Can you work these out from the model? Positions are in its coordinate system, mm. Face numbers are marked on the shaded views. Coordinates: 2 decimals unless noted, no trailing zeros. Loops run counter-clockwise (first coordinate to the right, second up) from the corner with the lowest first, then second, coordinate; pieces in that order, holes last. Notation, with made-up numbers: (61, -26) -> (95, -26) arc R32 cw to (95, 12) -> close; hole circle Ø9 at (39, -15). An arc over 180 degrees is marked (long way). Use one line per item in the form item = value. Start each with the question number.
(1) Imagine slicing it at A-A (z = 0). List the corners of the cut face in (x, y) for me.
(2) Imagine slicing it at C-C (y = -58). List the corners of the cut face in (x, z) for me.
(3) Thinking about a two-plate mould opening in Z: for the marked faces 1, 2, 3 and 4, which applies, released by +Z, released by -Z, zero draft, split by the parting line, or undercut?
(4) I need wall thicknesses on line 1 (Y direction, x = 4.5, z = -54); line 2 (Z direction, x = 8.25, y = -58); line 3 (Z direction, x = 14, y = -57). Which ranges of each line are inside material? Lowest first, please. Write a range as [from, to].
(5) I'm going to push flat-ended pins straight in: pin 1 (1 mm diameter, centred on x = 3, z = 16.5, fed in from +Y); pin 2 (20.5 mm diameter, centred on y = 51.27, z = -51.27, fed in from -X); pin 3 (4 mm diameter, centred on x = 14, z = -7, fed in from +Y); pin 4 (1 mm diameter, centred on x = 12.5, z = -45.5, fed in from -Y). Where does each tip first touch, or does it pass through?
(6) Imagine slicing it at D-D (x = 6.25). List the corners of the cut face in (y, z) for me.
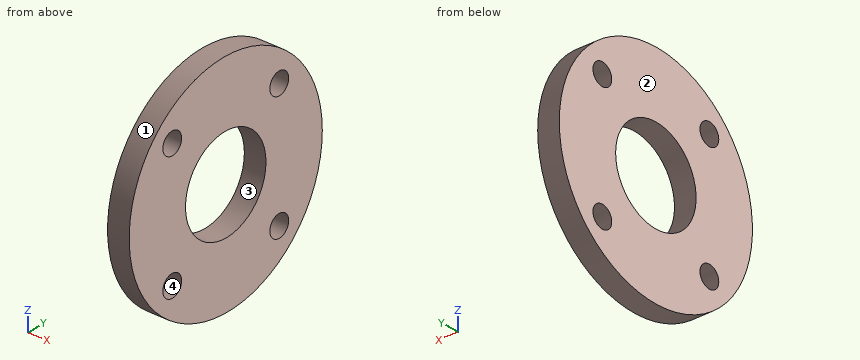
Autodesk Inventor part; units mm, degrees
ref_plane "YZ Plane" through (0, 0, 0) normal (1, 0, 0) x (0, 1, 0)
ref_plane "XZ Plane" through (0, 0, 0) normal (0, 1, 0) x (-1, 0, 0)
ref_plane "XY Plane" through (0, 0, 0) normal (0, 0, 1) x (1, 0, 0)
sketch "Sketch1" plane through (0, 0, 0) normal (0, 0, 1) x (1, 0, 0)
  line L0 (18, 92.5) -> (0, 92.5)
  line L1 (0, 92.5) -> (0, 38.55)
  line L2 (0, 38.55) -> (0, 0) construction
  line L3 (0, 0) -> (18, 0) construction
  line L4 (18, 92.5) -> (18, 38.55)
  line L5 (18, 38.55) -> (0, 38.55)
  line L6 (18, 38.55) -> (18, 0) construction
  dimension "d0" = 185
  dimension "d1" = 18
  dimension "d5" = 77.1
revolve "Revolution1" add sketch "Sketch1" angle 360 about axis through (0, 0, 0) along (1, 0, 0)
sketch "Sketch2" plane through (0, 0, 0) normal (-1, 0, 0) x (0, 0, 1)
  circle A0 centre (0, 0) radius 38.55
  line L0 (0, 72.5) -> (0, 0) construction
  circle A1 centre (0, 0) radius 92.5
  circle A2 centre (0, 0) radius 72.5 construction
  line L1 (0, 0) -> (51.2652, 51.2652) construction
  circle A3 centre (51.2652, 51.2652) radius 9
  dimension "d6" = 18
  dimension "d7" = 72.5
  dimension "d8" = 45
extrude "Extrusion1" cut sketch "Sketch2" against normal through all contours A3
pattern_circular "Circular Pattern1" count 4 over 360 about axis through (9, 0, 0) along (1, 0, 0) of "Extrusion1"
equation "\"d6\" = dd2"
equation "\"d7\" = 0.5 * k"
equation "\"d0\" = D"
equation "\"d1\" = b"
equation "\"d5\" = dd5"
equation "\"b\" = 18"
equation "\"D\" = 185"
equation "\"k\" = 145"
equation "\"dd2\" = 18"
equation "\"dd5\" = 77.1"
equation "\"Size_Designation\" = 1.2345"
properties part number "DIN 2576 Slip-On Flange for Welding Series 1 (ISO) - PN 10 65 x 76.1" material "Steel"
Worked out:
q1.outline = (0, -92.5) -> (18, -92.5) -> (18, -38.55) -> (0, -38.55) -> close; (0, 38.55) -> (18, 38.55) -> (18, 92.5) -> (0, 92.5) -> close
q2.outline = (0, -72.06) -> (18, -72.06) -> (18, -57.24) -> (0, -57.24) -> close; (0, -45.3) -> (18, -45.3) -> (18, 45.3) -> (0, 45.3) -> close; (0, 57.24) -> (18, 57.24) -> (18, 72.06) -> (0, 72.06) -> close
q3.face_1 = split by the parting line
q3.face_2 = zero draft
q3.face_3 = undercut
q3.face_4 = undercut
q4.line_1 = [-75.1, -59.84], [-42.69, 42.69], [59.84, 75.1]
q4.line_2 = [-72.06, -57.24], [-45.3, 45.3], [57.24, 72.06]
q4.line_3 = [-72.85, -58.2], [-44.33, 44.33], [58.2, 72.85]
q5.pin_1 = 91.11
q5.pin_2 = 0
q5.pin_3 = 92.36
q5.pin_4 = -80.82
q6.outline = circle Ø185 at (0, 0); hole circle Ø18 at (-51.27, -51.27); hole circle Ø18 at (-51.27, 51.27); hole circle Ø77.1 at (0, 0); hole circle Ø18 at (51.27, -51.27); hole circle Ø18 at (51.27, 51.27)
